```python
from build123d import *

# Parameters (mm, degrees)
SKETCH1_W           = 45.5
SKETCH1_H           = 10
SKETCH1_R           = 0.25
BOSS_EXTRUDE1_DEPTH = 6.5
SKETCH2_R           = 0.6
BOSS_EXTRUDE2_DEPTH = 5
SKETCH4_W           = 40
SKETCH4_H           = 2.5
CUT_EXTRUDE1_DEPTH  = 1
FILLET1_R           = 1


with BuildPart() as part:
    # Sketch1 → Boss-Extrude1 (new body)
    with BuildSketch(Plane(origin=(0, 0, 0), x_dir=(1, 0, 0), z_dir=(0, 1, 0))):
        Rectangle(SKETCH1_W, SKETCH1_H)
        with Locations(Location((-20.5, 0, 0), (0, 0, 270))):
            Circle(SKETCH1_R, mode=Mode.SUBTRACT)
        with Locations(Location((20.5, 0, 0), (0, 0, 270))):
            Circle(SKETCH1_R, mode=Mode.SUBTRACT)
    extrude(amount=BOSS_EXTRUDE1_DEPTH)

    # Sketch2 → Boss-Extrude2 (add)
    with BuildSketch(Plane.XZ):
        with Locations(Location((-21.75, 2, 0), (0, 0, 90))):
            Circle(SKETCH2_R)
        with Locations(Location((-21.75, -2, 0), (0, 0, 90))):
            Circle(SKETCH2_R)
        with Locations(Location((21.75, 2, 0), (0, 0, 90))):
            Circle(SKETCH2_R)
    extrude(amount=BOSS_EXTRUDE2_DEPTH)

    # Sketch4 → Cut-Extrude1 (cut)
    with BuildSketch(Plane(origin=(0, 6.5, 0), x_dir=(1, 0, 0), z_dir=(0, 1, 0))):
        Rectangle(SKETCH4_W, SKETCH4_H)
    extrude(amount=-CUT_EXTRUDE1_DEPTH, mode=Mode.SUBTRACT)

    # Fillet1
    fillet1_edges = [part.edges().sort_by_distance(p)[0] for p in [
        (22.75, 6.5, 0),
        (0, 6.5, -5),
        (-22.75, 6.5, 0),
        (0, 6.5, 5),
    ]]
    fillet(fillet1_edges, radius=FILLET1_R)


solid = part.part
```
Part model, mm, in its own coordinate system. A direction names the side the tool comes from. Give positions to 0.01 mm unless a question says otherwise; leave off trailing zeros. Loops run counter-clockwise (first coordinate to the right, second up) from the corner with the lowest first, then second, coordinate; pieces in that order, holes last. Notation, with made-up numbers: M -25,-18.5 L 5,-18.5 A16 cw 5,11.5 Z; hole C 38,24.5 d3. An arc over 180 degrees is marked long. Return JSON: item names as keys, results as strings.
1) Saw through at A-A, the plane x = -10. List the corners of the cut face in (y, z).
Calculated:
{"outline": "M 0,-5 L 5.5,-5 A1 ccw 6.5,-4 L 6.5,-1.25 L 5.5,-1.25 L 5.5,1.25 L 6.5,1.25 L 6.5,4 A1 ccw 5.5,5 L 0,5 Z"}
2) Drill centre lines: line 1 (X direction, y = 4.25, z = 0); line 2 (Z direction, x = 20.5, y = 2); line 3 (X direction, y = -0.75, z = 2). Where is each one in solid material? Low to high.
Calculated:
{"line 1": "x = -22.75 to -20.75, -20.25 to 20.25, 20.75 to 22.75", "line 2": "z = -5 to -0.25, 0.25 to 5", "line 3": "x = -22.35 to -21.15, 21.15 to 22.35"}
3) Pull direction X, two halves, no side cores. Call faces 4 (the face through (0, 6, -1.25)), 5 (the face through (0, 6.5, -2)), 6 (the face through (22.449, 6.215, -0.07)): released by +X, released by -X, zero draft, split by the parting line, or undercut.
Calculated:
{"face 4": "undercut", "face 5": "zero draft", "face 6": "released by +X"}
4) Flat gauge pins, fed straight in: pin 1 Ø4 at (x, z) = (-14, 0.5) entering from -Y; pin 2 Ø0.8 at (x, y) = (-5.5, 6) entering from -Z (3 decimals); pin 3 Ø4 at (x, y) = (1.5, -3.5) entering from -Z; pin 4 Ø2 at (x, z) = (5.5, 0) entering from +Y. Where does each tip first touch, or does it go through?
Calculated:
{"pin 1": "stops at y = 0", "pin 2": "stops at z = -4.995", "pin 3": "passes through", "pin 4": "stops at y = 5.5"}
5) Saw through at C-C, the plane z = -2. List the corners of the cut face in (x, y), then the cut area to 3 significant figures.
Calculated:
{"outline": "M -22.75,0 L -22.35,0 L -22.35,-5 L -21.15,-5 L -21.15,0 L 22.75,0 L 22.75,5.5 A1 ccw 21.75,6.5 L -21.75,6.5 A1 ccw -22.75,5.5 Z", "area": "301 mm2"}
6) Saw through at B-B, the plane z = 2. List the corners of the cut face in (x, y), then the cut area to 3 significant figures.
Calculated:
{"outline": "M -22.75,0 L -22.35,0 L -22.35,-5 L -21.15,-5 L -21.15,0 L 21.15,0 L 21.15,-5 L 22.35,-5 L 22.35,0 L 22.75,0 L 22.75,5.5 A1 ccw 21.75,6.5 L -21.75,6.5 A1 ccw -22.75,5.5 Z", "area": "307 mm2"}
7) 3-axis set-ups, long thin cutter, end or side, ignore diameter. For faces 1 (the face through (-22.345, -2.465, -2.078)), 2 (the face through (0, 5.5, 0)), 3 (the face through (22, -5, 2)): which of +Z, -Z, +X, -X, +Y, -Y reach the whole face in a straight line?
Calculated:
{"face 1": "-Y", "face 2": "+Y", "face 3": "+Z, -Z, +X, -X, -Y"}
